Geometry: final body of the model. Coordinates: model frame, mm. A direction names the side the tool comes from. Give positions to 0.01 mm unless a question says otherwise; leave off trailing zeros. Order: outer loops, then holes, each group sorted by start corner. A loop starts at its lowest first (then second) coordinate and runs counter-clockwise, first axis right, second up. Notation, with made-up numbers: (48, 63) -> (86, 63) arc R21 cw to (86, 80) -> close; hole circle Ø10 at (-20.5, 48.5). An arc over 180 degrees is marked (long way). One line per question, with ' | ' between items. Start each with the question number.
(1) Section D-D (z = -1.85). Return loops of the section in (x, y).
(2) Section A-A (y = 0). Return loops of the section in (x, z).
(3) Section B-B (x = 0.75). Return loops of the section in (y, z).
(4) Set-up query: faces 5 (the face through (0, -2.25, -2)), 6 (the face through (0, 2, 0)), 7 (the face through (5.5, 0, 0)), 8 (the face through (-5.85, 0.05, -1.99)), 9 (the face through (5.85, -0.05, -1.99)). Return all of +Z, -Z, +X, -X, +Y, -Y with unobstructed straight access to the full face (end or side cutting, diameter ignored); none if empty.
(5) Ray query, L1, parallel to Z at x = 0.25, y = 2.5; L2, parallel to Y at x = -2.5, z = 0.9; L3, parallel to X at y = 1.75, z = 2.1. Return the intervals inside material, ascending.
(6) First-contact query: pin 1 Ø1.1 at (x, z) = (1.5, -2) entering from -Y; pin 2 Ø1.5 at (x, z) = (1, -0.5) entering from +Y. Flat tips, straight axial feed; report the tip coordinate or a pass-through.
(7) Mould query, pull axis Z, two halves, no side actions, for faces 1 (the face through (0, 0, 3.5)), 2 (the face through (-9, 0, 2)), 3 (the face through (0, 0, -2.5)), 4 (the face through (0, -2, 0)). Classes: +Z half, -Z half, draft (parallel to the pull), parting line (faces both ways), or undercut.
(8) Section C-C (z = 0.1). Return loops of the section in (x, y), then the cut area to 3 significant figures.
```python
from build123d import *

# Parameters (mm, degrees)
BOSS_EXTRU_1_DEPTH = 1.5
BOSS_EXTRU_2_START = 1.5
BOSS_EXTRU_2_DEPTH = 2
BOSS_EXTRU_3_DEPTH = 1


with BuildPart() as part:
    # Esquisse1 → Boss.-Extru.1 (new, symmetric)
    with BuildSketch(Plane.XY):
        with BuildLine():
            Line((-3.5, 2), (3.5, 2))
            ThreePointArc((3.5, 2), (5.5, 0), (3.5, -2))
            Line((3.5, -2), (-3.5, -2))
            ThreePointArc((-3.5, -2), (-5.5, 0), (-3.5, 2))
        make_face()
    extrude(amount=BOSS_EXTRU_1_DEPTH, both=True)

    # Esquisse2 → Boss.-Extru.2 (add)
    with BuildSketch(Plane.XY.offset(BOSS_EXTRU_2_START)):
        with BuildLine():
            Line((-5, 4), (5, 4))
            ThreePointArc((5, 4), (9, 0), (5, -4))
            Line((5, -4), (-5, -4))
            ThreePointArc((-5, -4), (-9, 0), (-5, 4))
        make_face()
    extrude(amount=BOSS_EXTRU_2_DEPTH)

    # Esquisse3 → Boss.-Extru.3 (add)
    with BuildSketch(Plane(origin=(0, 0, -1.5), x_dir=(-1, 0, 0), z_dir=(0, 0, -1))):
        with BuildLine():
            Line((-3.6, 2.25), (3.6, 2.25))
            ThreePointArc((3.6, 2.25), (5.85, 0), (3.6, -2.25))
            Line((3.6, -2.25), (-3.6, -2.25))
            ThreePointArc((-3.6, -2.25), (-5.85, 0), (-3.6, 2.25))
        make_face()
    extrude(amount=BOSS_EXTRU_3_DEPTH)


solid = part.part
```
Response:
1) outline: (-3.6, -2.25) -> (3.6, -2.25) arc R2.25 ccw to (3.6, 2.25) -> (-3.6, 2.25) arc R2.25 ccw to start
2) outline: (-9, 1.5) -> (-5.5, 1.5) -> (-5.5, -1.5) -> (-5.85, -1.5) -> (-5.85, -2.5) -> (5.85, -2.5) -> (5.85, -1.5) -> (5.5, -1.5) -> (5.5, 1.5) -> (9, 1.5) -> (9, 3.5) -> (-9, 3.5) -> close
3) outline: (-4, 1.5) -> (-2, 1.5) -> (-2, -1.5) -> (-2.25, -1.5) -> (-2.25, -2.5) -> (2.25, -2.5) -> (2.25, -1.5) -> (2, -1.5) -> (2, 1.5) -> (4, 1.5) -> (4, 3.5) -> (-4, 3.5) -> close
4) face 5: -Z, +X, -X, -Y | face 6: +X, -X, +Y | face 7: +X | face 8: -Z, -X | face 9: -Z, +X
5) L1: z = 1.5 to 3.5 | L2: y = -2 to 2 | L3: x = -8.6 to 8.6
6) pin 1: stops at y = -2.25 | pin 2: stops at y = 2
7) face 1: +Z half | face 2: draft | face 3: -Z half | face 4: undercut
8) outline: (-3.5, -2) -> (3.5, -2) arc R2 ccw to (3.5, 2) -> (-3.5, 2) arc R2 ccw to start | area: 40.6 mm^2
